Read the model definition and answer for the solid it produces. Units are mm, in the model's axes. A direction names the side the tool comes from. Give positions to 0.01 mm unless a question says otherwise; leave off trailing zeros. Loops run counter-clockwise (first coordinate to the right, second up) from the corner with the lowest first, then second, coordinate; pieces in that order, holes last. Notation, with made-up numbers: (45.5, 19) - (93.5, 19) arc R26 ccw to (93.5, 51) - close; hole circle Ø5 at (-10.5, 79.5). An arc over 180 degrees is marked (long way). Use a Markdown table: item, result. Add a question column.
Item 1: Consider probe 1 along X at (y, z) = (1.8, 28); probe 2 along X at (y, z) = (0.7, 12); probe 3 along X at (y, z) = (4.8, 46). Determine where each line is inside the solid, lowest interval first. Write a range as [from, to].
Item 2: A cutting plane is placed at A-A (y = 1.65). Determine the outline of the cut face in (x, z).
Item 3: Each of these flat-tipped pins is pushed along its axis until it touches: P1, Ø2.5, axis at x = 32, y = 2, coming from the +Z side; P2, Ø1.5, axis at x = -36, y = 4.5, coming from the +Z side; P3, Ø2.5, axis at y = 1.5, z = 12, coming from the -X side; P4, Ø12, axis at x = -14, z = 55, coming from the +Y side. Where does it stop, or does it pass through?
Item 4: A cutting plane is placed at D-D (x = -1). Determine the outline of the cut face in (y, z).
Item 5: Which of the six approach directions +Z, -Z, +X, -X, +Y, -Y give full straight-line access (tool end or side, diameter ignored) to faces 4 (the face through (-45, 2, 61)), 5 (the face through (17.5, 2, 13)), 6 (the face through (24.755, 2.535, 7.139))?
Item 6: A cutting plane is placed at C-C (z = 36.5). Determine the outline of the cut face in (x, y).
Item 7: For a pull along X with two mould halves and no side action, classify faces 1 (the face through (-44.342, 2.535, 2.086)), 2 (the face through (22.5, 2, 32)), 3 (the face through (11, 5, 30)) as +X half, -X half, draft (parallel to the pull), parting line (faces both ways), or undercut.
Item 8: A cutting plane is placed at B-B (z = 23.5). Determine the outline of the cut face in (x, y).
Solid Edge part; units mm, degrees
sketch "Sketch1" plane through (0, 0, 0) normal (0, -1, 0) x (1, 0, 0)
  line L0 (-43, 61) -> (-43, 5)
  line L1 (-22.5, 5) -> (-43, 5)
  line L2 (-22.5, 52.7379) -> (-22.5, 5)
  line L3 (22.5, 52.7379) -> (-22.5, 52.7379)
  line L4 (22.5, 5) -> (22.5, 52.7379)
  line L5 (43, 5) -> (22.5, 5)
  line L6 (43, 61) -> (43, 5)
  line L7 (47.75, 61) -> (43, 61)
  line L8 (46.5, 0) -> (47.75, 61)
  line L9 (17.5, 0) -> (46.5, 0)
  line L10 (17.5, 25) -> (17.5, 0)
  line L11 (-17.5, 25) -> (17.5, 25)
  line L12 (-17.5, 0) -> (-17.5, 25)
  line L13 (-46.5, 0) -> (-17.5, 0)
  line L14 (-46.5, 0) -> (-47.75, 61)
  line L15 (-47.75, 61) -> (-43, 61)
extrude "Protrusion1" add sketch "Sketch1" against normal blind 5
fillet "Round_1" radius 7.5 6 edges at (-46.5, 2.5, 0) (46.5, 2.5, 0) (43, 2.5, 5) (-43, 2.5, 5) (-22.5, 2.5, 5) (22.5, 2.5, 5)
Geometry says:
| question | item | result |
|---|---|---|
| 1 | probe 1 | [-47.07, -43], [-22.5, 22.5], [43, 47.07] |
| 1 | probe 2 | [-46.75, -42.98], [-22.52, -17.5], [17.5, 22.52], [42.98, 46.75] |
| 1 | probe 3 | [-47.44, -43], [-22.5, 22.5], [43, 47.44] |
| 2 | outline | (-47.75, 61) - (-46.65, 7.35) arc R7.5 ccw to (-39.15, 0) - (-17.5, 0) - (-17.5, 25) - (17.5, 25) - (17.5, 0) - (39.15, 0) arc R7.5 ccw to (46.65, 7.35) - (47.75, 61) - (43, 61) - (43, 12.5) arc R7.5 cw to (35.5, 5) - (30, 5) arc R7.5 cw to (22.5, 12.5) - (22.5, 52.74) - (-22.5, 52.74) - (-22.5, 12.5) arc R7.5 cw to (-30, 5) - (-35.5, 5) arc R7.5 cw to (-43, 12.5) - (-43, 61) - close |
| 3 | P1 | z = 5 |
| 3 | P2 | z = 5.1 |
| 3 | P3 | x = -46.77 |
| 3 | P4 | y = 5 |
| 4 | outline | (0, 25) - (5, 25) - (5, 52.74) - (0, 52.74) - close |
| 5 | face 4 | +Z, +X, -X, +Y, -Y |
| 5 | face 5 | -Z, +Y, -Y |
| 5 | face 6 | +Z, +Y, -Y |
| 6 | outline | (-47.25, 0) - (-43, 0) - (-43, 5) - (-47.25, 5) - close; (-22.5, 0) - (22.5, 0) - (22.5, 5) - (-22.5, 5) - close; (43, 0) - (47.25, 0) - (47.25, 5) - (43, 5) - close |
| 7 | face 1 | -X half |
| 7 | face 2 | undercut |
| 7 | face 3 | draft |
| 8 | outline | (-46.98, 0) - (-43, 0) - (-43, 5) - (-46.98, 5) - close; (-22.5, 0) - (-17.5, 0) - (-17.5, 5) - (-22.5, 5) - close; (17.5, 0) - (22.5, 0) - (22.5, 5) - (17.5, 5) - close; (43, 0) - (46.98, 0) - (46.98, 5) - (43, 5) - close |
